Answer from the drawing. Dimensions are ordinates in mm from the lowest x, y and z of the part. A direction names the side the tool comes from. Give positions to 0.01 mm unless a question says otherwise; leave off trailing zeros. Write each loop counter-clockwise with the first axis right and the second up, starting at its lowest first coordinate (ties: lowest second). Pieces come first, ordered by that corner, then holes. Notation, with made-up numbers: M -21.5,16 L 4.5,16 A25 cw 4.5,28 Z; hole C -27,77 d1. An arc over 180 degrees is marked long. Answer as a JSON object with one key per item and string values.
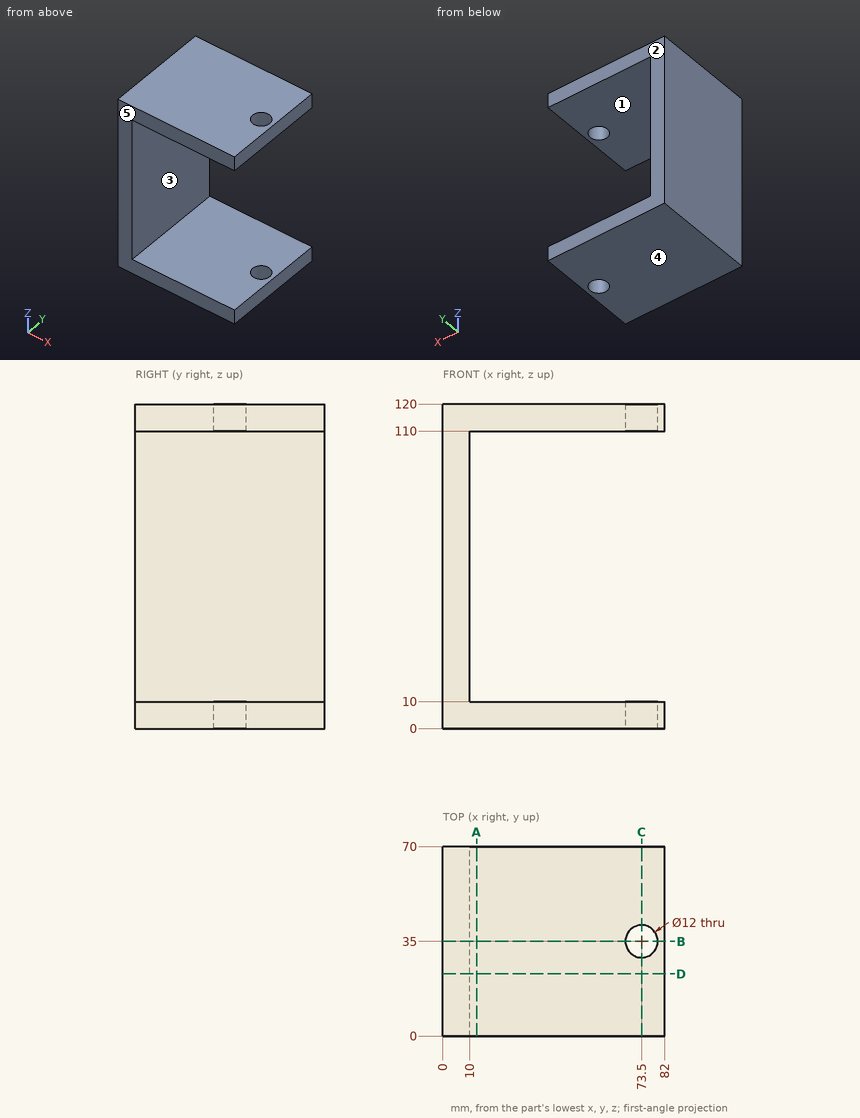
1. A cutting plane is placed at B-B, the plane y = 35. Give the vertices of the cut face in (x, z).
Verdict:
{"outline": "M 0,0 L 67.5,0 L 67.5,10 L 10,10 L 10,110 L 67.5,110 L 67.5,120 L 0,120 Z; M 79.5,0 L 82,0 L 82,10 L 79.5,10 Z; M 79.5,110 L 82,110 L 82,120 L 79.5,120 Z"}
2. A cutting plane is placed at D-D, the plane y = 23. Give the vertices of the cut face in (x, z), plus the area to 3 significant figures.
Verdict:
{"outline": "M 0,0 L 82,0 L 82,10 L 10,10 L 10,110 L 82,110 L 82,120 L 0,120 Z", "area": "2,640 mm2"}
3. A cutting plane is placed at C-C, the plane x = 73.5. Give the vertices of the cut face in (y, z).
Verdict:
{"outline": "M 0,0 L 29,0 L 29,10 L 0,10 Z; M 0,110 L 29,110 L 29,120 L 0,120 Z; M 41,0 L 70,0 L 70,10 L 41,10 Z; M 41,110 L 70,110 L 70,120 L 41,120 Z"}
4. Consider line 1 along Y through (x, z) = (73.5, 113.25); line 2 along X through (y, z) = (35, 114); line 3 along Z through (x, y) = (48.5, 22.5). Determine where each line is inside the solid, lowest interval first.
Verdict:
{"line 1": "y = 0 to 29, 41 to 70", "line 2": "x = 0 to 67.5, 79.5 to 82", "line 3": "z = 0 to 10, 110 to 120"}
5. For the marked faces 1 and 2, determine the directions among +Z, -Z, +X, -X, +Y, -Y from which every point of the face is accessible in a straight line to the end or side of a thin tool.
Verdict:
{"face 1": "+X, +Y, -Y", "face 2": "+Z, -Z, +X, -X, +Y"}
6. A flat-ended cylindrical pin translates along its axis: pin 1 (21 mm diameter, centred on y = 39.5, z = 74, fed in from +X). Find the tip coordinate at first contact, or state that the pin passes through.
Verdict:
{"pin 1": "stops at x = 10"}
7. The mould has two halves that part along Z. Classify the marked faces 3, 4 and 5: released by +Z, released by -Z, zero draft, split by the parting line, or undercut.
Verdict:
{"face 3": "undercut", "face 4": "released by -Z", "face 5": "zero draft"}
8. A cutting plane is placed at A-A, the plane x = 12.5. Give the vertices of the cut face in (y, z), plus the area to 3 significant figures.
Verdict:
{"outline": "M 0,0 L 70,0 L 70,10 L 0,10 Z; M 0,110 L 70,110 L 70,120 L 0,120 Z", "area": "1,400 mm2"}
